For this review, use the dimensioned drawing (mm, ordinates from the lowest corner) and the shaded views. A direction names the side the tool comes from. Round coordinates to 2 decimals unless told otherwise and drop trailing zeros. Write each loop counter-clockwise with the first axis right and the second up, starting at its lowest first coordinate (ties: lowest second). Pieces come first, ordered by that corner, then holes. Notation, with made-up numbers: M 77,75 L 86,75 A25 ccw 86,87 Z; hole C 52,59.5 d1. An arc over 180 degrees is marked long. Use one line per item in the form item = value. Start each with the question number.
Item 1: Add section C-C (x = 24.5). Count the separate pieces of the cut face and the enclosed holes in it, and give its area (3 significant figures).
Item 2: For P1, Ø9.5, axis at x = 24.5, z = 24.5, coming from the +Y side; P2, Ø5.5, axis at y = 89.5, z = 34.5, coming from the +X side; P3, Ø2.5, axis at y = 107, z = 16, coming from the -X side; P4, Ø8, axis at x = 7, y = 35, coming from the +Z side, all flat-tipped, find the tip position at first contact; note any pin that passes through.
Item 3: For line 1 (Y direction, x = 24, z = 16); line 2 (Y direction, x = 24.85, z = 33); line 3 (Y direction, x = 24.5, z = 13), list the stretches that pass through material, from the lowest coordinate up. Write a range as [from, to].
Item 4: For the marked faces 1 and 2, list the 3-axis set-ups (+Z, -Z, +X, -X, +Y, -Y) from which the entire face can be reached by the end or side of a thin tool; tool diameter is ignored.
Item 5: Draft analysis for pull direction Z (two halves, no side actions). For the marked faces 3, 4 and 5, state which applies: released by +Z, released by -Z, zero draft, split by the parting line, or undercut.
Item 6: Add section B-B (y = 94.5). State the section outline as (x, z) points.
Item 7: Add section A-A (y = 30.57). State the section outline as (x, z) points.
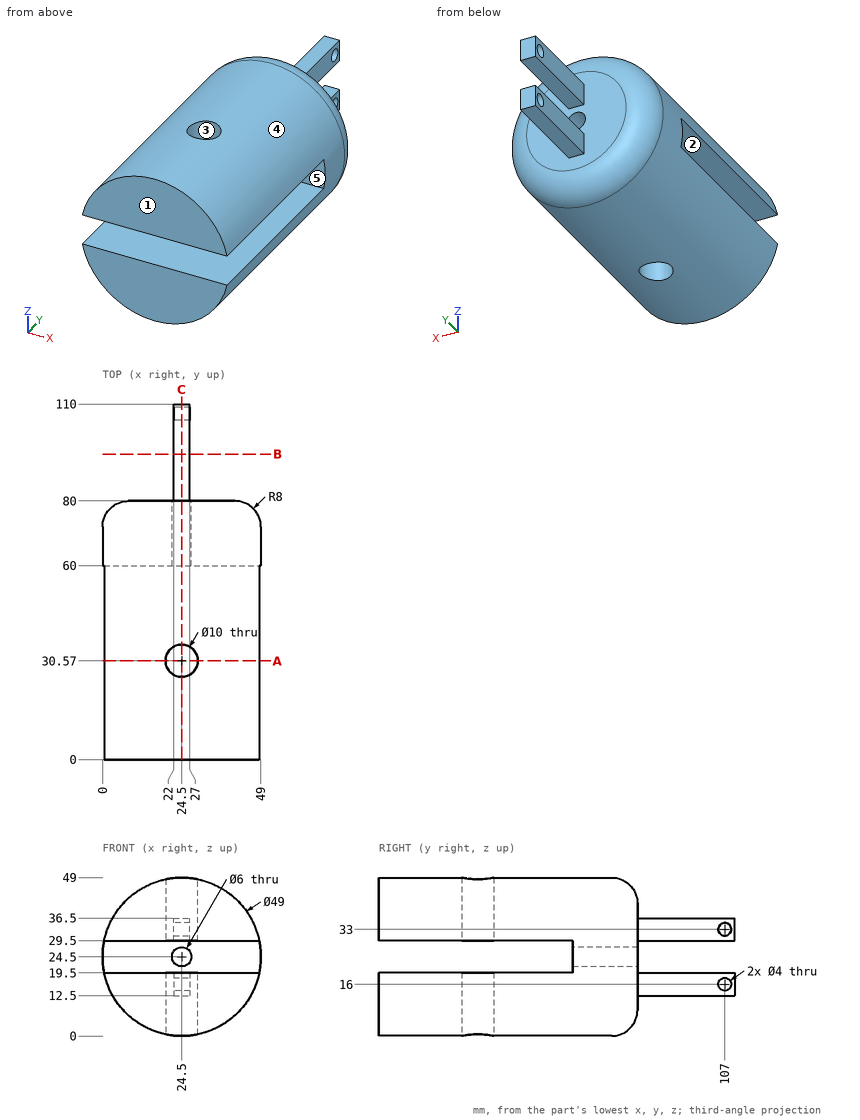
Calculated:
q1.separate_pieces = 4
q1.enclosed_holes = 2
q1.area = 3,180 mm^2
q2.P1 = 80
q2.P2 = 27
q2.P3 = through
q2.P4 = 44.95
q3.line_1 = [0, 25.6], [35.54, 105], [109, 110]
q3.line_2 = [0, 25.58], [35.56, 105], [109, 110]
q3.line_3 = [0, 25.57], [35.57, 110]
q4.face_1 = +Z, -Z, +X, -X, -Y
q4.face_2 = +X, -X, -Y
q5.face_3 = zero draft
q5.face_4 = split by the parting line
q5.face_5 = undercut
q6.outline = M 22,12.5 L 27,12.5 L 27,19.5 L 22,19.5 Z; M 22,29.5 L 27,29.5 L 27,36.5 L 22,36.5 Z
q7.outline = M 0.52,19.5 A24.5 ccw 19.5,0.52 L 19.5,19.5 Z; M 0.52,29.5 L 19.5,29.5 L 19.5,48.48 A24.5 ccw Z; M 29.5,0.52 A24.5 ccw 48.48,19.5 L 29.5,19.5 Z; M 29.5,29.5 L 48.48,29.5 A24.5 ccw 29.5,48.48 Z
